from build123d import *

# Parameters (mm, degrees)
PAD_DEPTH       = 10
SKETCH001_R     = 1.375
POCKET_DEPTH    = 10
PAD001_DEPTH    = 33
SKETCH003_R     = 1.375
POCKET001_DEPTH = 10
SKETCH004_R     = 1.375
POCKET002_DEPTH = 10
FILLET_1_R      = 9
FILLET_2_R      = 6
CHAMFER_SIZE    = 5
CHAMFER001_SIZE = 0.5
CHAMFER002_SIZE = 0.5


with BuildPart() as part:
    # Sketch → Pad (new body, symmetric)
    with BuildSketch(Plane.YZ):
        Polygon((4, 4), (17, 4), (17, 18), (54, 18), (54, -15), (51, -15), (51, 15), (20, 15), (20, -15), (12, -15), (12, -4), (4, -4), align=None)
    extrude(amount=PAD_DEPTH, both=True)

    # Sketch001 → Pocket (cut)
    with BuildSketch(Plane(origin=(0, 4, 0), x_dir=(0, 0, -1), z_dir=(0, -1, 0))):
        Circle(SKETCH001_R)
    extrude(amount=-POCKET_DEPTH, mode=Mode.SUBTRACT)

    # Sketch002 → Pad001 (new body)
    with BuildSketch(Plane(origin=(0, 0, 18), x_dir=(0, -1, 0), z_dir=(0, 0, 1))):
        with BuildLine():
            ThreePointArc((-58.492889, 1.949289), (-59, 0), (-58.492889, -1.949289))
            Line((-54, -10), (-58.492889, -1.949289))
            Line((-54, 10), (-54, -10))
            Line((-58.492889, 1.949289), (-54, 10))
        make_face()
    extrude(amount=-PAD001_DEPTH)

    # Sketch003 → Pocket001 (cut)
    with BuildSketch(Plane(origin=(0, 0, 18), x_dir=(0, -1, 0), z_dir=(0, 0, 1))):
        with Locations((-55, 0)):
            Circle(SKETCH003_R)
    extrude(amount=-POCKET001_DEPTH, mode=Mode.SUBTRACT)

    # Sketch004 → Pocket002 (cut)
    with BuildSketch(Plane.YX.offset(15)):
        with Locations((55, 0)):
            Circle(SKETCH004_R)
        with Locations((16, 0)):
            Circle(SKETCH004_R)
    extrude(amount=-POCKET002_DEPTH, mode=Mode.SUBTRACT)

    # Fillet 1
    fillet_1_edges = [part.edges().sort_by_distance(p)[0] for p in [
        (0, 17, 18),
    ]]
    fillet(fillet_1_edges, radius=FILLET_1_R)

    # Fillet 2
    fillet_2_edges = [part.edges().sort_by_distance(p)[0] for p in [
        (0, 20, 15),
        (0, 51, 15),
    ]]
    fillet(fillet_2_edges, radius=FILLET_2_R)

    # Chamfer
    chamfer_edges = [part.edges().sort_by_distance(p)[0] for p in [
        (-10, 52.5, -15),
        (-10, 16, -15),
        (10, 52.5, -15),
        (10, 16, -15),
    ]]
    chamfer(chamfer_edges, length=CHAMFER_SIZE)

    # Chamfer001
    chamfer001_edges = [part.edges().sort_by_distance(p)[0] for p in [
        (0, 56.375, 18),
        (0, 4, 1.375),
        (0, 53.625, -15),
        (0, 14.625, -15),
    ]]
    chamfer(chamfer001_edges, length=CHAMFER001_SIZE)

    # Chamfer002
    chamfer002_edges = [part.edges().sort_by_distance(p)[0] for p in [
        (-10, 40, 18),
        (-10, 51, -0.5),
        (-10, 19.636039, 15.363961),
        (-10, 49.242641, 13.242641),
        (-10, 17, 6.5),
        (-10, 35.5, 15),
        (-10, 10.5, 4),
        (-10, 21.757359, 13.242641),
        (-10, 4, 0),
        (-10, 20, -0.5),
        (-10, 8, -4),
        (-10, 12, -7),
    ]]
    chamfer(chamfer002_edges, length=CHAMFER002_SIZE)


solid = part.part
Read the model definition and answer for the solid it produces. Units are mm, in the model's axes. A direction names the side the tool comes from. Round coordinates to 2 decimals unless told otherwise and drop trailing zeros. Write each loop counter-clockwise with the first axis right and the second up, starting at its lowest first coordinate (ties: lowest second). Pieces come first, ordered by that corner, then holes. Notation, with made-up numbers: (-22.5, -10.5) - (18.5, -10.5) arc R17 ccw to (18.5, -3.5) - close; hole circle Ø3 at (-6, 3.5). An arc over 180 degrees is marked (long way). Use a Markdown table: item, result.
(1) Straight lines are drawn through the part: line 1 along X through (y, z) = (6.5, 0) (3 decimals); line 2 along Z through (x, y) = (4, 37.5); line 3 along Y through (x, z) = (4.75, 13.5). For each, find the intervals that lie inside material, in ascending order. Write a range as [from, to].
Reported:
| item | result |
|---|---|
| line 1 | [-10, -1.375], [1.375, 10] |
| line 2 | [15, 18] |
| line 3 | [18.21, 22.03], [48.97, 56.93] |
(2) Each of these flat-tipped pins is pushed along its axis until it touches: pin 1 Ø2 at (x, z) = (-7, 2.5) entering from +Y; pin 2 Ø1 at (x, z) = (6, 10.5) entering from +Y; pin 3 Ø0.8 at (x, y) = (0, 55) entering from +Z; pin 4 Ø8 at (y, z) = (25, 0.5) entering from -X. Where does it stop, or does it pass through?
Reported:
| item | result |
|---|---|
| pin 1 | y = 56.23 |
| pin 2 | y = 56.51 |
| pin 3 | z = 8 |
| pin 4 | through |
(3) The part is cut by section B-B (y = 11). Write down the section's boundary in (x, z) (3 decimals).
Reported:
| item | result |
|---|---|
| outline | (-10, -3.5) - (-9.5, -4) - (10, -4) - (10, 4) - (-9.5, 4) - (-10, 3.5) - close; hole circle Ø2.75 at (0, 0) |
(4) Which of the six approach directions +Z, -Z, +X, -X, +Y, -Y give full straight-line access (tool end or side, diameter ignored) to faces 1 (the flat face through (0, 51, -3)), 2 (the cylindrical face through (0.06, 14.626, -9.817)), 3 (the flat face through (0, 12, -10)), 4 (the conical face through (-9.64, 49.39, 13.29)), 5 (the flat face through (3, 4, 0))?
Reported:
| item | result |
|---|---|
| face 1 | -Z, +X, -X |
| face 2 | -Z |
| face 3 | -Z, +X, -X, -Y |
| face 4 | -Z, -X |
| face 5 | +Z, -Z, +X, -X, -Y |
(5) The part is cut by section C-C (x = 2.5). Write down the section's boundary in (y, z), then the cut area to 3 significant figures.
Reported:
| item | result |
|---|---|
| outline | (4, -4) - (12, -4) - (12, -15) - (20, -15) - (20, 9) arc R6 cw to (26, 15) - (45, 15) arc R6 cw to (51, 9) - (51, -15) - (58.19, -15) - (58.19, 18) - (26, 18) arc R9 ccw to (17, 9) - (17, 4) - (4, 4) - close |
| area | 586 mm2 |
(6) The part is cut by section D-D (y = 55). Write down the section's boundary in (x, z) (3 decimals), then the cut area to 3 significant figures.
Reported:
| item | result |
|---|---|
| outline | (-8.208, -11.792) - (-5, -15) - (-1.875, -15) - (-1.375, -14.5) - (-1.375, -5) - (1.375, -5) - (1.375, -14.5) - (1.875, -15) - (5, -15) - (8.208, -11.792) - (8.208, 18) - (1.875, 18) - (1.375, 17.5) - (1.375, 8) - (-1.375, 8) - (-1.375, 17.5) - (-1.875, 18) - (-8.208, 18) - close |
| area | 476 mm2 |
(7) The part is cut by section A-A (z = 0). Write down the section's boundary in (x, y) (3 decimals).
Reported:
| item | result |
|---|---|
| outline | (-10, 4.5) - (-9.5, 4) - (-1.875, 4) - (-1.375, 4.5) - (-1.375, 14) - (1.375, 14) - (1.375, 4.5) - (1.875, 4) - (10, 4) - (10, 20) - (-9.5, 20) - (-10, 19.5) - close; (-10, 51.5) - (-9.5, 51) - (10, 51) - (10, 54) - (1.949, 58.493) arc R4 ccw to (-1.949, 58.493) - (-10, 54) - close |
(8) The mould has two halves that part along Z. Classify faces 6 (the flat face through (0, 20, -3)), 7 (the flat face through (-8, 16, -12)), 8 (the flat face through (0, 14, 0)), 9 (the conical face through (-9.865, 19.827, 15.039)): released by +Z, released by -Z, zero draft, split by the parting line, or undercut.
Reported:
| item | result |
|---|---|
| face 6 | zero draft |
| face 7 | released by -Z |
| face 8 | undercut |
| face 9 | released by +Z |
